Verification items for this drawing (mm, ordinates from the low corner). Round coordinates to 2 decimals unless told otherwise and drop trailing zeros. Write each loop counter-clockwise with the first axis right and the second up, starting at its lowest first coordinate (ties: lowest second). Pieces come first, ordered by that corner, then holes.
Item 1: Cross-section at B-B (y = 27). Enter the section's corners in (x, z).
Item 2: Cross-section at A-A (z = 4.1). Enter the section's corners in (x, y).
Item 3: Depth check by flat-ended pin: P1, Ø1.5, axis at x = 18.5, z = 3, coming from the -Y side. Enter the tip coordinate at first touch or a pass-through.
Item 4: Scan lines: probe 1 along X at (y, z) = (21.5, 1.8); probe 2 along X at (y, z) = (23.5, 2.5). Record each from-to range of solid material in increasing order.
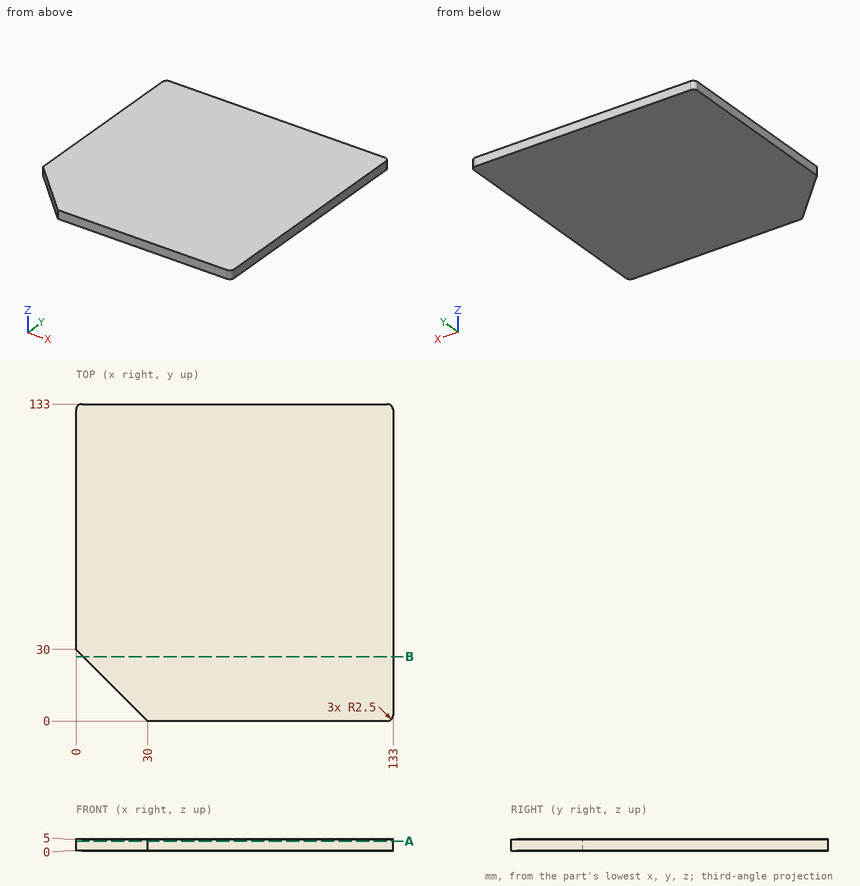
Resolved:
1. outline: (3, 0) - (133, 0) - (133, 5) - (3, 5) - close
2. outline: (0, 30) - (30, 0) - (130.5, 0) arc R2.5 ccw to (133, 2.5) - (133, 130.5) arc R2.5 ccw to (130.5, 133) - (2.5, 133) arc R2.5 ccw to (0, 130.5) - close
3. P1: stops at y = 10.75
4. probe 1: x = 8.5 to 133
4. probe 2: x = 6.5 to 133
